from build123d import *

# Parameters (mm, degrees)
BOSS_EXTRUDE1_DEPTH = 19.05
FILLET1_R           = 2.2225
SKETCH2_R           = 2.413
CUT_EXTRUDE1_DEPTH  = 272.420720469
SKETCH3_R           = 4.445
CUT_EXTRUDE2_DEPTH  = 6.35


with BuildPart() as part:
    # Sketch1 → Boss-Extrude1 (new body)
    with BuildSketch(Plane(origin=(0, 0, 0), x_dir=(1, 0, 0), z_dir=(0, 1, 0))):
        with BuildLine():
            Line((0, 171.45), (190.5, 171.45))
            Line((190.5, 171.45), (190.5, 158.75))
            ThreePointArc((190.5, 158.75), (187.325, 155.575), (190.5, 152.4))
            Line((190.5, 152.4), (209.55, 152.4))
            Line((209.55, 152.4), (209.55, 133.35))
            Line((209.55, 133.35), (190.5, 133.35))
            ThreePointArc((190.5, 133.35), (187.325, 130.175), (190.5, 127))
            Line((190.5, 127), (190.5, 82.55))
            ThreePointArc((190.5, 82.55), (187.325, 79.375), (190.5, 76.2))
            Line((190.5, 76.2), (209.55, 76.2))
            Line((209.55, 76.2), (209.55, 57.15))
            Line((209.55, 57.15), (191.092301163, 57.15))
            ThreePointArc((191.092301163, 57.15), (187.931266017, 54.272458919), (190.5, 50.855736572))
            Line((190.5, 50.855736572), (190.5, 0))
            Line((190.5, 0), (139.7, 0))
            Line((139.7, 0), (139.7, 19.05))
            Line((139.7, 19.05), (50.8, 19.05))
            Line((50.8, 19.05), (50.8, 0))
            Line((50.8, 0), (0, 0))
            Line((0, 0), (0, 12.7))
            ThreePointArc((0, 12.7), (3.175, 15.875), (0, 19.05))
            Line((0, 19.05), (-19.05, 19.05))
            Line((-19.05, 19.05), (-19.05, 38.1))
            Line((-19.05, 38.1), (0, 38.1))
            ThreePointArc((0, 38.1), (3.175, 41.275), (0, 44.45))
            Line((0, 44.45), (0, 88.9))
            ThreePointArc((0, 88.9), (3.175, 92.075), (0, 95.25))
            Line((0, 95.25), (-19.05, 95.25))
            Line((-19.05, 95.25), (-19.05, 114.3))
            Line((-19.05, 114.3), (0, 114.3))
            ThreePointArc((0, 114.3), (3.175, 117.475), (0, 120.65))
            Line((0, 120.65), (0, 171.45))
        make_face()
    extrude(amount=BOSS_EXTRUDE1_DEPTH)

    # Fillet1
    fillet1_edges = [part.edges().sort_by_distance(p)[0] for p in [
        (139.7, 9.525, 0),
        (139.7, 9.525, -19.05),
        (50.8, 9.525, -19.05),
        (50.8, 9.525, 0),
    ]]
    fillet(fillet1_edges, radius=FILLET1_R)

    # Sketch2 → Cut-Extrude1 (cut, through all)
    with BuildSketch(Plane.XZ):
        with Locations(Location((95.25, -31.75, 0), (0, 0, 270))):
            Circle(SKETCH2_R)
        with Locations(Location((95.25, -50.8, 0), (0, 0, 270))):
            Circle(SKETCH2_R)
    extrude(amount=-CUT_EXTRUDE1_DEPTH, mode=Mode.SUBTRACT)

    # Sketch3 → Cut-Extrude2 (cut)
    with BuildSketch(Plane(origin=(0, 19.05, 0), x_dir=(1, 0, 0), z_dir=(0, 1, 0))):
        with Locations(Location((95.25, 31.75, 0), (0, 0, 270))):
            Circle(SKETCH3_R)
        with Locations(Location((95.25, 50.8, 0), (0, 0, 270))):
            Circle(SKETCH3_R)
    extrude(amount=-CUT_EXTRUDE2_DEPTH, mode=Mode.SUBTRACT)


solid = part.part
Design review of the part built by this model. Coordinates are the model's own, in mm. A direction names the side the tool comes from. Coordinates: 2 decimals unless noted, no trailing zeros. Order: outer loops, then holes, each group sorted by start corner. A loop starts at its lowest first (then second) coordinate and runs counter-clockwise, first axis right, second up. Notation, with made-up numbers: (61, 55) -> (118, 55) arc R18 ccw to (118, 78) -> close; hole circle Ø1 at (29.25, -14.5). An arc over 180 degrees is marked (long way). Use one line per item in the form item = value. Start each with the question number.
(1) For faces 5 (the flat face through (200, 9, -57.15)), 6 (the flat face through (190.5, 9, -165)), 7 (the cylindrical face through (92.55, 15.92, -54.33)), 8 (the flat face through (-9, 9, -19.05)), list the 3-axis set-ups (+Z, -Z, +X, -X, +Y, -Y) from which the entire face can be reached by the end or side of a thin tool; tool diameter is ignored.
(2) Add section D-D on y = 6. Give the number of separate pieces and of enclosed holes in the cut face, plus the area to 3 significant figures.
(3) Add section A-A on z = -31.75. State the section outline as (x, y) points (3 decimals).
(4) Insertion check: pin 1 (5.5 mm diameter, centred on x = 79, y = 7.5, fed in from +Z); pin 2 (9.5 mm diameter, centred on x = 197, y = 6, fed in from +Z); pin 3 (10 mm diameter, centred on y = 7.5, z = -163, fed in from +X). Each pin has a flat end and moves straight along its axis. Give the tip position at first contact, or say it passes through.
(5) For probe 1 along X at (y, z) = (17.25, -31.5); probe 2 along Z at (x, y) = (95, 17); probe 3 along X at (y, z) = (6.5, -50.8), list the stretches that pass through material, from the lowest coordinate up.
(6) The part is to be moulded in two halves that separate along X. For faces 1 (the flat face through (0, 9, -146)), 2 (the flat face through (190.5, 9, -26)), 3 (the flat face through (-9, 9, -95.25)), 4 (the flat face through (93, 12.7, -30)), say which applies: +X half, -X half, draft (parallel to the pull), parting line (faces both ways), or undercut.
(7) Add section B-B on x = 95.25. State the section outline as (y, z) points (3 decimals), plus the area to 3 significant figures.
(8) Add section C-C on z = -147. State the section outline as (x, y) points, plus the area to 3 significant figures.
Answer block:
q1.face_5 = +Z, +X, +Y, -Y
q1.face_6 = -Z, +X, +Y, -Y
q1.face_7 = +Y
q1.face_8 = +Z, -X, +Y, -Y
q2.separate_pieces = 1
q2.enclosed_holes = 2
q2.area = 32,300 mm²
q3.outline = (-19.05, 0) -> (92.837, 0) -> (92.837, 12.7) -> (90.805, 12.7) -> (90.805, 19.05) -> (-19.05, 19.05) -> close; (97.663, 0) -> (190.5, 0) -> (190.5, 19.05) -> (99.695, 19.05) -> (99.695, 12.7) -> (97.663, 12.7) -> close
q4.pin_1 = -19.05
q4.pin_2 = -57.15
q4.pin_3 = 190.5
q5.probe_1 = -19.05 to 90.81, 99.69 to 190.5
q5.probe_2 = -171.45 to -55.24, -46.36 to -36.19, -27.31 to -19.05
q5.probe_3 = 0 to 92.84, 97.66 to 190.5
q6.face_1 = -X half
q6.face_2 = +X half
q6.face_3 = draft
q6.face_4 = undercut
q7.outline = (0, -171.45) -> (19.05, -171.45) -> (19.05, -55.245) -> (12.7, -55.245) -> (12.7, -53.213) -> (0, -53.213) -> close; (0, -48.387) -> (12.7, -48.387) -> (12.7, -46.355) -> (19.05, -46.355) -> (19.05, -36.195) -> (12.7, -36.195) -> (12.7, -34.163) -> (0, -34.163) -> close; (0, -29.337) -> (12.7, -29.337) -> (12.7, -27.305) -> (19.05, -27.305) -> (19.05, -19.05) -> (0, -19.05) -> close
q7.area = 2,670 mm²
q8.outline = (0, 0) -> (209.55, 0) -> (209.55, 19.05) -> (0, 19.05) -> close
q8.area = 3,990 mm²
